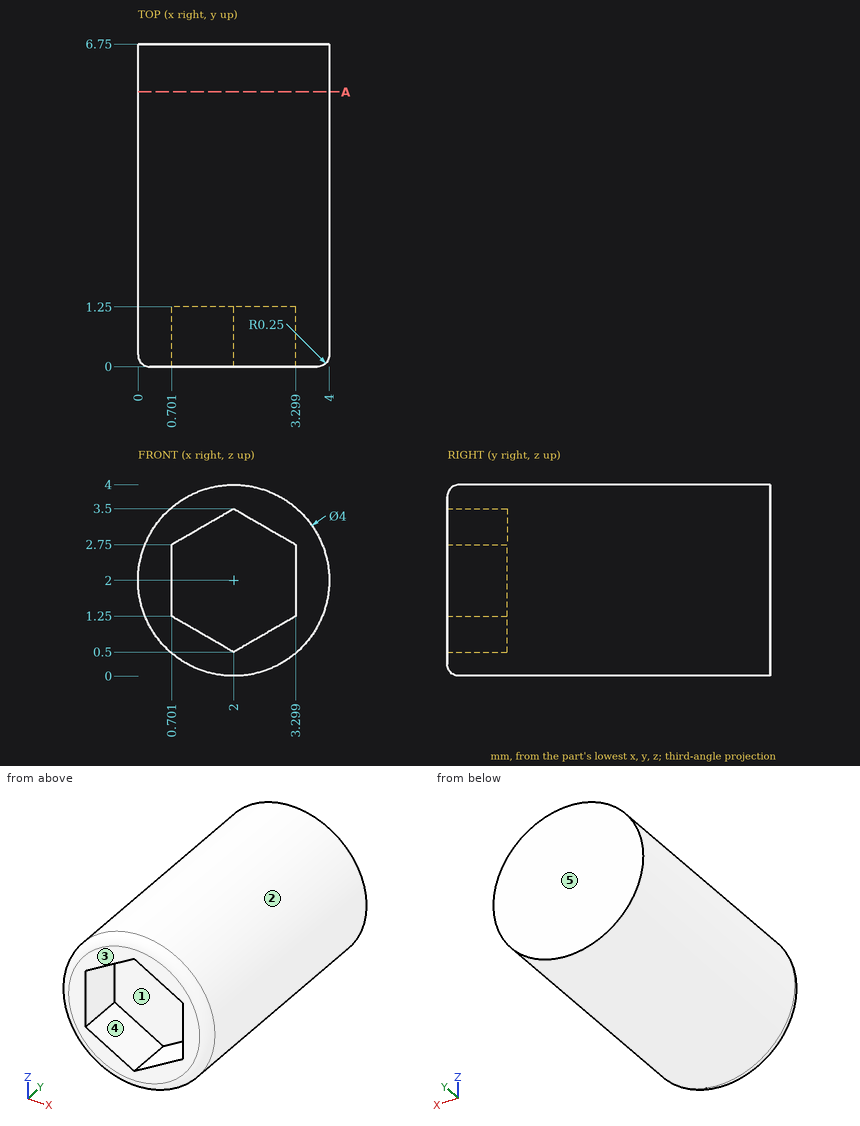
Can you work these out from the drawing? Everything is in mm from the part's minimum corner. A direction names the side the tool comes from. Coordinates: 2 decimals unless noted, no trailing zeros. Order: outer loops, then holes, each group sorted by start corner. A loop starts at its lowest first (then second) coordinate and runs counter-clockwise, first axis right, second up. Notation, with made-up numbers: (13, 66.5) -> (72, 66.5) arc R22 ccw to (72, 100.5) -> close; hole circle Ø1 at (29.25, -17). An arc over 180 degrees is marked (long way). Return JSON: item names as keys, results as strings.
1) On a 3-axis mill with a long thin cutter (end or side, diameter ignored), from which of +Z, -Z, +X, -X, +Y, -Y can I reach the whole of each face in a straight line? I mean the marked faces 4 and 5. Say none if no direction works.
Conclusion:
{"face 4": "-Y", "face 5": "+Z, -Z, +X, -X, +Y"}
2) If I drill on probe 1 along Y at (x, z) = (2, 2.25); probe 2 along X at (y, z) = (1.5, 1.7); probe 3 along X at (y, z) = (5.75, 0.3), over which ranges is the centre line in solid material (lowest first)?
Conclusion:
{"probe 1": "y = 1.25 to 6.75", "probe 2": "x = 0.02 to 3.98", "probe 3": "x = 0.95 to 3.05"}
3) Thinking about a two-plate mould opening in Z: for the marked faces 1, 2 and 3, which applies, +Z half, -Z half, draft (parallel to the pull), parting line (faces both ways), or undercut?
Conclusion:
{"face 1": "undercut", "face 2": "parting line", "face 3": "draft"}
4) If we section it at A-A on y = 5.75: List the corners of the cut face in (x, z) for me, plus the area to 3 significant figures.
Conclusion:
{"outline": "circle Ø4 at (2, 2)", "area": "12.6 mm²"}
5) I'm going to push a flat-ended pin straight in: P1, Ø1.3, axis at x = 2.5, z = 2, coming from the -Y side. Where does the tip first touch, or does it pass through?
Conclusion:
{"P1": "stops at y = 1.25"}
